Read the model definition and answer for the solid it produces. Units are mm, in the model's axes. A direction names the side the tool comes from. Give positions to 0.01 mm unless a question says otherwise; leave off trailing zeros. Order: outer loops, then holes, each group sorted by start corner. A loop starts at its lowest first (then second) coordinate and runs counter-clockwise, first axis right, second up. Notation, with made-up numbers: (65.5, -0.75) - (108.5, -0.75) arc R20 cw to (108.5, 12.25) - close; hole circle Ø9 at (25, 29.25). An arc over 180 degrees is marked (long way). Answer as CSV lines item,"result". Start each with the question number.
from build123d import *

# Parameters (mm, degrees)
SKETCH_1_R               = 27.5
EXTRUDE_5_DEPTH          = 6
SKETCH_8_R               = 30
EXTRUDE_6_DEPTH          = 2
EXTRUDE_START            = 2
SKETCH_9_R               = 30
EXTRUDE_7_DEPTH          = 2
CUT_EXTRUDE_1_DEPTH      = 44.588989435
CUT_EXTRUDE_1_DEPTH_BACK = 44.588989435
SKETCH_12_R              = 2.11
SKETCH_12_R_2            = 2.1


with BuildPart() as part:
    # Эскиз1 → Бобышка-Вытянуть5 (new body)
    with BuildSketch(Plane(origin=(0, 0, 0), x_dir=(1, 0, 0), z_dir=(0, 1, 0))):
        with Locations(Location((0, 0, 0), (0, 0, 270))):
            Circle(SKETCH_1_R)
    extrude(amount=EXTRUDE_5_DEPTH)

    # Эскиз8 → Бобышка-Вытянуть6 (add)
    with BuildSketch(Plane(origin=(0, 6, 0), x_dir=(1, 0, 0), z_dir=(0, 1, 0))):
        with Locations(Location((0, 0, 0), (0, 0, 270))):
            Circle(SKETCH_8_R)
    extrude(amount=EXTRUDE_6_DEPTH)

    # Эскиз9 → Бобышка-Вытянуть7 (add)
    with BuildSketch(Plane.XZ.offset(EXTRUDE_START)):
        with Locations(Location((0, 0, 0), (0, 0, 90))):
            Circle(SKETCH_9_R)
    extrude(amount=-EXTRUDE_7_DEPTH)

    # Эскиз12 → Вырез-Вытянуть1 (cut, two sides: drawn at the far end of the back side and taken through both)
    with BuildSketch(Plane(origin=(0, 8, 0), x_dir=(1, 0, 0), z_dir=(0, 1, 0)).offset(-CUT_EXTRUDE_1_DEPTH_BACK)):
        with Locations(Location((14.095522252, -2.742507282, 0), (0, 0, 270))):
            Circle(SKETCH_12_R)
        with Locations(Location((1.726848044, -14.255633609, 0), (0, 0, 270))):
            Circle(SKETCH_12_R_2)
        with Locations(Location((-14.100702431, 2.71574754, 0), (0, 0, 270))):
            Circle(SKETCH_12_R_2)
        with Locations(Location((-1.699786223, 14.25888567, 0), (0, 0, 270))):
            Circle(SKETCH_12_R_2)
    extrude(amount=CUT_EXTRUDE_1_DEPTH + CUT_EXTRUDE_1_DEPTH_BACK, mode=Mode.SUBTRACT)


solid = part.part
(1) Section B-B, the plane y = -1 is taken. Write down the section's boundary in (x, z), and give its area (3 significant figures).
(2) Which of the six approach directions +Z, -Z, +X, -X, +Y, -Y give full straight-line access (tool end or side, diameter ignored) to faces 4 (the flat face through (0, 8, 0)), 5 (the flat face through (-24.3, 6, 13.2))?
(3) Section D-D, the plane z = 20 is taken. Write down the section's boundary in (x, y).
(4) Determine the mould class of faces 1 (the cylindrical face through (1.32, 6.99, -29.97)), 2 (the flat face through (0, -2, 0)), 3 (the cylindrical face through (1.819, 2.93, 12.158)) for opening direction X: released by +X, released by -X, zero draft, split by the parting line, or undercut.
(5) Flat-ended cylindrical pins translate along their axes: pin 1 Ø3 at (x, y) = (-23.5, 0) entering from +Z; pin 2 Ø5 at (x, z) = (14.1, 2.74) entering from +Y; pin 3 Ø3 at (y, z) = (5.5, -21) entering from -X; pin 4 Ø4 at (x, z) = (-14.1, -2.72) entering from +Y. Find the tip coordinate at first contact, or state that the pin passes through.
(6) Straight lines are drawn through the part: line 1 (Y direction, x = -23.5, z = -14.5); line 2 (X direction, y = 4.75, z = -15); line 3 (Z direction, x = 0.5, y = 5). For each, find the intervals that lie inside material, in ascending order. Write a range as [from, to].
(7) Section C-C, the plane x = -5.5 is taken. Write down the section's boundary in (y, z), and give its area (3 significant figures).
(8) Section A-A, the plane z = -2.5 is taken. Write down the section's boundary in (x, y).
Checks:
1,outline,"circle Ø60 at (0, 0); hole circle Ø4.2 at (-14.1, -2.72); hole circle Ø4.2 at (-1.7, -14.26); hole circle Ø4.2 at (1.73, 14.26); hole circle Ø4.22 at (14.1, 2.74)"
1,area,"2,770 mm²"
2,face 4,"+Z, -Z, +X, -X, +Y"
2,face 5,"none"
3,outline,"(-22.36, -2) - (22.36, -2) - (22.36, 0) - (18.87, 0) - (18.87, 6) - (22.36, 6) - (22.36, 8) - (-22.36, 8) - (-22.36, 6) - (-18.87, 6) - (-18.87, 0) - (-22.36, 0) - close"
4,face 1,"split by the parting line"
4,face 2,"zero draft"
4,face 3,"undercut"
5,pin 1,"stops at z = 20.4"
5,pin 2,"stops at y = 8"
5,pin 3,"stops at x = -22.72"
5,pin 4,"passes through"
6,line 1,"y = [-2, 0], [6, 8]"
6,line 2,"x = [-23.05, -3.66], [0.27, 23.05]"
6,line 3,"z = [-27.5, 12.55], [15.96, 27.5]"
7,outline,"(-2, -29.49) - (0, -29.49) - (0, -26.94) - (6, -26.94) - (6, -29.49) - (8, -29.49) - (8, 29.49) - (6, 29.49) - (6, 26.94) - (0, 26.94) - (0, 29.49) - (-2, 29.49) - close"
7,area,"559 mm²"
8,outline,"(-29.9, -2) - (-16.19, -2) - (-16.19, 8) - (-29.9, 8) - (-29.9, 6) - (-27.39, 6) - (-27.39, 0) - (-29.9, 0) - close; (-12.01, -2) - (29.9, -2) - (29.9, 0) - (27.39, 0) - (27.39, 6) - (29.9, 6) - (29.9, 8) - (-12.01, 8) - close"
